```python
from build123d import *

# Parameters (mm, degrees)
F1_DEPTH = 23
F2_R     = 1.5
F3_DEPTH = 4
F4_R     = 1.5
F5_DEPTH = 4


with BuildPart() as f1:
    # F0 (on Top) → F1 (new body)
    with BuildSketch(Plane.XY):
        Polygon((-1.356773, -2.35), (1.356773, -2.35), (2.713546, 0), (1.356773, 2.35), (-1.356773, 2.35), (-2.713546, 0), align=None)
    extrude(amount=F1_DEPTH)

    # F2 (on face) → F3 (cut)
    with BuildSketch(Plane.XY.offset(23)):
        Circle(F2_R)
    extrude(amount=-F3_DEPTH, mode=Mode.SUBTRACT)

    # F4 (on face) → F5 (cut)
    with BuildSketch(Plane(origin=(0, 0, 0), x_dir=(1, 0, 0), z_dir=(0, 0, -1))):
        Circle(F4_R)
    extrude(amount=-F5_DEPTH, mode=Mode.SUBTRACT)


solid = f1.part
```
Input: part model. Units: mm. Frame: model coordinates. A direction names the side the tool comes from. Give positions to 0.01 mm unless a question says otherwise; leave off trailing zeros. Order: outer loops, then holes, each group sorted by start corner. A loop starts at its lowest first (then second) coordinate and runs counter-clockwise, first axis right, second up. Notation, with made-up numbers: M 32.25,89.5 L 53.25,89.5 A26 cw 53.25,106.5 Z; hole C 66,58 d5. An arc over 180 degrees is marked long. Return JSON: item names as keys, results as strings.
Item 1: Access query for faces 1 (the cylindrical face through (-1.5, 0.07, 21.03)), 2 (the cylindrical face through (-1.5, -0.07, 1.97)), 3 (the flat face through (-2.026, 1.191, 11.339)). Directions: +Z, -Z, +X, -X, +Y, -Y. A direction counts if a zero-diameter tool reaches every point of the face in a straight line with its end or side. Return the directions, or none.
Solutions:
{"face 1": "+Z", "face 2": "-Z", "face 3": "+Z, -Z, -X, +Y"}
Item 2: Cut plane C-C (y = 0.25). Return loops of the section in (x, z), then the cut area to 3 significant figures.
Solutions:
{"outline": "M -2.57,0 L -1.48,0 L -1.48,4 L 1.48,4 L 1.48,0 L 2.57,0 L 2.57,23 L 1.48,23 L 1.48,19 L -1.48,19 L -1.48,23 L -2.57,23 Z", "area": "94.5 mm^2"}
Item 3: First-contact query: P1, Ø2.5, axis at x = 0, y = 0, coming from the -Z side. Flat tip, straight axial feed; report the tip coordinate or a pass-through.
Solutions:
{"P1": "z = 4"}
Item 4: Cut plane D-D (z = 10.75). Return loops of the section in (x, y).
Solutions:
{"outline": "M -2.71,0 L -1.36,-2.35 L 1.36,-2.35 L 2.71,0 L 1.36,2.35 L -1.36,2.35 Z"}
Item 5: Pull-direction query (Y, two-part tool) for faces 4 (the flat face through (0, 2, 0)), 5 (the flat face through (2.045, 1.159, 11.339)), 6 (the flat face through (0, 0, 4)); classes: +Y half, -Y half, draft (parallel to the pull), parting line (faces both ways), or undercut.
Solutions:
{"face 4": "draft", "face 5": "+Y half", "face 6": "undercut"}
Item 6: Ray query, probe 1 along Y at (x, z) = (0, 2.2); probe 2 along Z at (x, y) = (0, 0.5); probe 3 along X at (y, z) = (0.05, 1.75). Return the intervals inside material, ascending.
Solutions:
{"probe 1": "-2.35 to -1.5, 1.5 to 2.35", "probe 2": "4 to 19", "probe 3": "-2.68 to -1.5, 1.5 to 2.68"}
Item 7: Cut plane B-B (x = 0). Return loops of the section in (y, z), then the cut area to 3 significant figures.
Solutions:
{"outline": "M -2.35,0 L -1.5,0 L -1.5,4 L 1.5,4 L 1.5,0 L 2.35,0 L 2.35,23 L 1.5,23 L 1.5,19 L -1.5,19 L -1.5,23 L -2.35,23 Z", "area": "84.1 mm^2"}
Item 8: Cut plane A-A (z = 2). Return loops of the section in (x, y).
Solutions:
{"outline": "M -2.71,0 L -1.36,-2.35 L 1.36,-2.35 L 2.71,0 L 1.36,2.35 L -1.36,2.35 Z; hole C 0,0 d3"}
